Geometry check sheet. Reference: the model listing, model coordinates, mm. A direction names the side the tool comes from. Give positions to 0.01 mm unless a question says otherwise; leave off trailing zeros. Write each loop counter-clockwise with the first axis right and the second up, starting at its lowest first coordinate (ties: lowest second). Pieces come first, ordered by that corner, then holes. Notation, with made-up numbers: (63, -27) -> (92, -27) arc R30 ccw to (92, 6) -> close; hole circle Ø6 at (-8.75, -11.5). An arc over 180 degrees is marked (long way). One line per item, written item: value.
from build123d import *

# Parameters (mm, degrees)
SKETCH117_W             = 40
SKETCH117_H             = 30
SKETCH117_R             = 10
PAD021_DEPTH            = 3
SKETCH118_W             = 35
SKETCH118_H             = 25
SKETCH118_W_2           = 33
SKETCH118_H_2           = 23
PAD022_DEPTH            = 3
FILLET013_R             = 5
FILLET014_R             = 1.5
FILLET016_R             = 2.5
PAD023_DEPTH            = 2.5
SKETCH121_W             = 5
SKETCH121_H             = 3
POCKET043_DEPTH         = 37.501
CHAMFER002_SIZE         = 2
SKETCH122_W             = 24
SKETCH122_H             = 3
POCKET044_DEPTH         = 27.501
CHAMFER003_SIZE         = 1
BODY010_PLACEMENT_ANGLE = 20


with BuildPart() as part:
    # Sketch117 → Pad021 (new body)
    with BuildSketch(Plane.XY):
        Rectangle(SKETCH117_W, SKETCH117_H)
        Circle(SKETCH117_R, mode=Mode.SUBTRACT)
    extrude(amount=PAD021_DEPTH)

    # Sketch118 (on Face7 of Pad021) → Pad022 (join)
    with BuildSketch(Plane.XY.offset(3)):
        Rectangle(SKETCH118_W, SKETCH118_H)
        Rectangle(SKETCH118_W_2, SKETCH118_H_2, mode=Mode.SUBTRACT)
    extrude(amount=PAD022_DEPTH)

    # Fillet013
    fillet013_edges = [part.edges().sort_by_distance(p)[0] for p in [
        (20, -15, 1.5),
        (20, 15, 1.5),
        (-20, 15, 1.5),
        (-20, -15, 1.5),
    ]]
    fillet(fillet013_edges, radius=FILLET013_R)

    # Fillet014
    fillet014_edges = [part.edges().sort_by_distance(p)[0] for p in [
        (16.5, 11.5, 4.5),
        (16.5, -11.5, 4.5),
        (-16.5, -11.5, 4.5),
        (-16.5, 11.5, 4.5),
    ]]
    fillet(fillet014_edges, radius=FILLET014_R)

    # Fillet016
    fillet016_edges = [part.edges().sort_by_distance(p)[0] for p in [
        (-17.5, -12.5, 4.5),
        (-17.5, 12.5, 4.5),
        (17.5, 12.5, 4.5),
        (17.5, -12.5, 4.5),
    ]]
    fillet(fillet016_edges, radius=FILLET016_R)

    # Sketch119 (on Face14 of Fillet014) → Pad023 (join, symmetric)
    with BuildSketch(Plane(origin=(0, 0, 0), x_dir=(-1, 0, 0), z_dir=(0, 1, 0))):
        Polygon((15, 3), (17.5, 3), (17.5, 7), (18.5, 7), (18.5, 8), (17, 9), (15, 9), align=None)
    pad023 = extrude(amount=PAD023_DEPTH, both=True)

    # Mirrored003: Pad023 across Sketch119 V_Axis
    add(pad023.mirror(Plane(origin=(0, 0, 0), x_dir=(0, 1, 0), z_dir=(-1, 0, 0))))

    # Sketch121 (on Face5 of Mirrored003) → Pocket043 (cut, through all)
    with BuildSketch(Plane(origin=(-17.5, 0, 0), x_dir=(0, -1, 0), z_dir=(-1, 0, 0))):
        with Locations((-5, 4.5)):
            Rectangle(SKETCH121_W, SKETCH121_H)
        with Locations((5, 4.5)):
            Rectangle(SKETCH121_W, SKETCH121_H)
    extrude(amount=-POCKET043_DEPTH, mode=Mode.SUBTRACT)

    # Chamfer002
    chamfer002_edges = [part.edges().sort_by_distance(p)[0] for p in [
        (-16.25, -2.5, 3),
        (-15, 0, 3),
        (-16.25, 2.5, 3),
        (16.25, 2.5, 3),
        (15, 0, 3),
        (16.25, -2.5, 3),
    ]]
    chamfer(chamfer002_edges, length=CHAMFER002_SIZE)

    # Sketch122 (on Face36 of Chamfer002) → Pocket044 (cut, through all)
    with BuildSketch(Plane(origin=(0, 12.5, 0), x_dir=(-1, 0, 0), z_dir=(0, 1, 0))):
        with Locations((0, 4.5)):
            Rectangle(SKETCH122_W, SKETCH122_H)
    extrude(amount=-POCKET044_DEPTH, mode=Mode.SUBTRACT)

    # Chamfer003
    chamfer003_edges = [part.edges().sort_by_distance(p)[0] for p in [
        (0, 15, 0),
    ]]
    chamfer(chamfer003_edges, length=CHAMFER003_SIZE)


with BuildPart() as part_1:
    # Body010 placement: moved
    add(part.part.moved(Location((-357.518507, 122.858339, 205.085809))).rotate(Axis((-357.518507, 122.858339, 205.085809), (1, 0, 0)), BODY010_PLACEMENT_ANGLE))


solid = part_1.part
1) Scan lines: probe 1 along X at (y, z) = (118, 211.25); probe 2 along X at (y, z) = (119.75, 211.25); probe 3 along Z at (x, y) = (-358, 109.75). Record each from-to range of solid material in increasing order.
Verdict:
probe 1: -376.02 to -372.52, -342.52 to -339.02
probe 2: -375.02 to -372.52, -342.52 to -340.02
probe 3: 200.31 to 203.51
2) Tool access check on faces 1 (the cylindrical face through (-340.77, 132.388, 213.366)), 2 (the flat face through (-341.559, 131.606, 214.655)), 3 (the flat face through (-375.019, 113, 206)), 4 (the flat face through (-344.04, 110.52, 205.36)). Record the directions out of +Z, -Z, +X, -X, +Y, -Y that give a thin tool (end or side, any length) a straight path to the whole face; none if there is none.
Verdict:
face 1: +Z, +X
face 2: +Z, +X, -X
face 3: +Z, -X, -Y
face 4: +Z
3) Sectioned sample at A-A on x = -365. Record the cut outline in (y, z), plus the area to 3 significant figures.
Verdict:
outline: (107.74, 202.77) -> (108.42, 200.9) -> (109.7, 200.3) -> (116.62, 202.82) -> (115.6, 205.64) -> close; (128.07, 210.17) -> (129.09, 207.36) -> (136.01, 209.87) -> (136.61, 211.16) -> (135.93, 213.04) -> close
area: 49.2 mm^2
4) Mould release check, pull along Y, two halves, no side actions. Record for faces 5 (the flat face through (-376.019, 120, 212)), 6 (the cylindrical face through (-341.47, 131.72, 213.12)), 7 (the flat face through (-341.8, 118.193, 207.63)), 8 (the conical face through (-339.522, 135.036, 209.821)): released by +Y, released by -Y, zero draft, split by the parting line, or undercut.
Verdict:
face 5: zero draft
face 6: undercut
face 7: undercut
face 8: released by +Y
5) Depth check by flat-ended pin: pin 1 Ø2.5 at (y, z) = (113, 207) entering from -X; pin 2 Ø1.6 at (y, z) = (120.5, 212) entering from +X; pin 3 Ø5 at (y, z) = (115, 205.5) entering from +X; pin 4 Ø12 at (x, y) = (-372.5, 113.5) entering from +Z. Enter the tip coordinate at first touch or a pass-through.
Verdict:
pin 1: x = -375.02
pin 2: x = -339.02
pin 3: x = -337.52
pin 4: z = 213.44
6) Sectioned sample at C-C on x = -356.5. Record the cut outline in (y, z).
Verdict:
outline: (107.74, 202.77) -> (108.42, 200.9) -> (109.7, 200.3) -> (113.51, 201.68) -> (112.48, 204.5) -> close; (131.18, 211.31) -> (132.21, 208.49) -> (136.01, 209.87) -> (136.61, 211.16) -> (135.93, 213.04) -> close
7) Sectioned sample at B-B on x = -347. Record the cut outline in (y, z), plus the area to 3 significant figures.
Verdict:
outline: (107.74, 202.77) -> (108.42, 200.9) -> (109.7, 200.3) -> (136.01, 209.87) -> (136.61, 211.16) -> (135.93, 213.04) -> close
area: 89.0 mm^2
